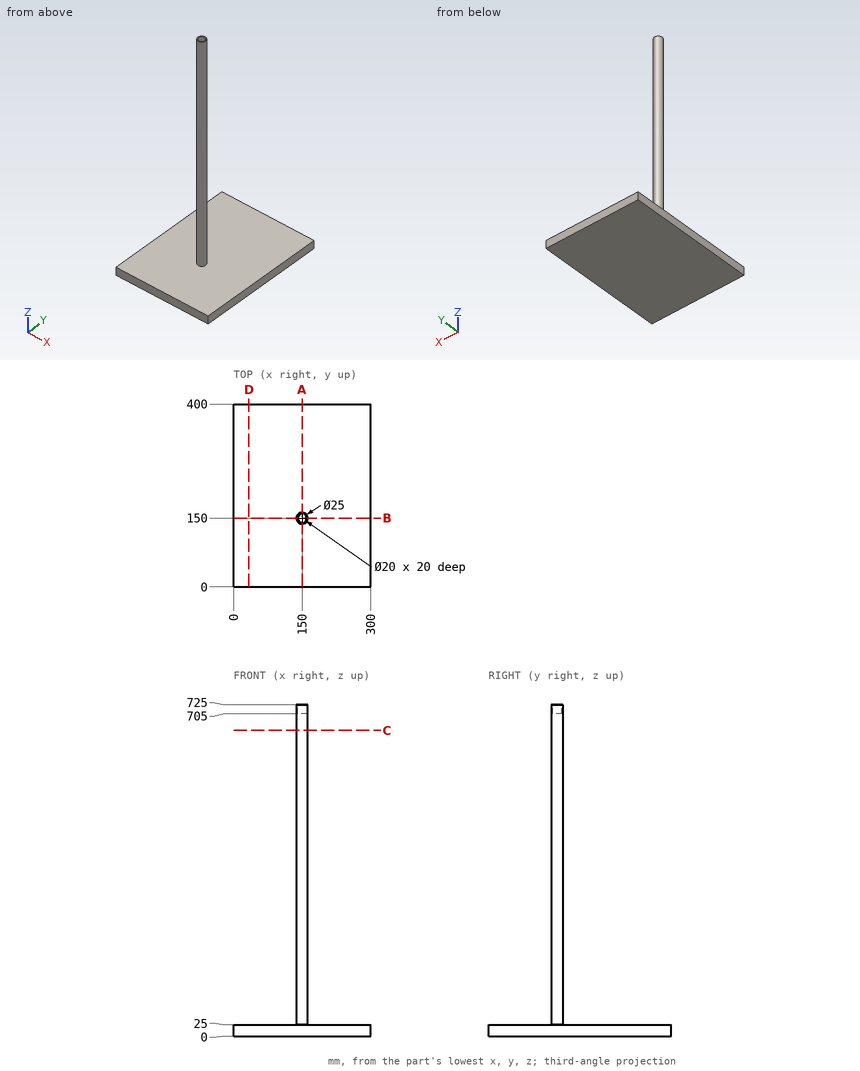
Part print with two shaded views. Sizes in mm from the minimum x, y, z corner. Round coordinates to 2 decimals unless told otherwise and drop trailing zeros. Loops run counter-clockwise (first coordinate to the right, second up) from the corner with the lowest first, then second, coordinate; pieces in that order, holes last.
Item 1: Saw through at A-A (x = 150). List the corners of the cut face in (y, z), then the cut area to 3 significant figures.
Item 2: Saw through at C-C (z = 669). List the corners of the cut face in (x, y), then the cut area to 3 significant figures.
Item 3: Saw through at D-D (x = 33.5). List the corners of the cut face in (y, z), then the cut area to 3 significant figures.
Item 4: Pin check, flat tip, straight feed: P1, Ø1, axis at x = 187.5, y = 334, coming from the +Z side. Stop position of the tip, or through.
Item 5: Saw through at B-B (y = 150). List the corners of the cut face in (x, z).
Item 6: Drill centre lines: line 1 along Y through (x, z) = (150, 710); line 2 along Z through (x, y) = (161, 291.5); line 3 along Y through (x, z) = (159.5, 314.5). Where is each one in solid material? Low to high.
Worked answers:
1. outline: (0, 0) - (400, 0) - (400, 25) - (162.5, 25) - (162.5, 725) - (160, 725) - (160, 705) - (140, 705) - (140, 725) - (137.5, 725) - (137.5, 25) - (0, 25) - close
1. area: 27,100 mm2
2. outline: circle Ø25 at (150, 150)
2. area: 491 mm2
3. outline: (0, 0) - (400, 0) - (400, 25) - (0, 25) - close
3. area: 10,000 mm2
4. P1: stops at z = 25
5. outline: (0, 0) - (300, 0) - (300, 25) - (162.5, 25) - (162.5, 725) - (160, 725) - (160, 705) - (140, 705) - (140, 725) - (137.5, 725) - (137.5, 25) - (0, 25) - close
6. line 1: y = 137.5 to 140, 160 to 162.5
6. line 2: z = 0 to 25
6. line 3: y = 141.88 to 158.12
